Model file for the job. Use its own axes, mm. Give positions to 0.01 mm unless a question says otherwise; leave off trailing zeros. Loops run counter-clockwise (first coordinate to the right, second up) from the corner with the lowest first, then second, coordinate; pieces in that order, holes last. Notation, with made-up numbers: M 86,-12.5 L 90,-12.5 A30 ccw 90,18.5 Z; hole C -18,-1.5 d10. An arc over 180 degrees is marked long. Use CSV: the item, a comma, the result in double quotes. Start each with the question number.
(1) Slice it at C-C on y = 33.5. List the corners of the cut face in (x, z).
(2) Slice it at A-A on z = -55. List the corners of the cut face in (x, y).
(3) Flat gauge pins, fed straight in: P1, Ø4, axis at y = 39.24, z = 66.83, coming from the +X side; P2, Ø1, axis at x = 1, y = -15, coming from the -Z side; P3, Ø1, axis at x = -0.5, z = 19.5, coming from the -Y side; P4, Ø0.8, axis at x = 0, y = -22.5, coming from the +Z side. Where does each tip first touch, or does it go through?
(4) Slice it at B-B on x = 0.4. State how many separate pieces and enclosed holes the cut face has, and give its area (3 significant figures).
(5) Wall check: line 1 along Z through (x, y) = (0.5, 0); line 2 along Y through (x, z) = (-0.75, 0); line 3 along Y through (x, z) = (0.1, -22.5). Give the ranges that are in metal, low to high. Write a range as from..to.
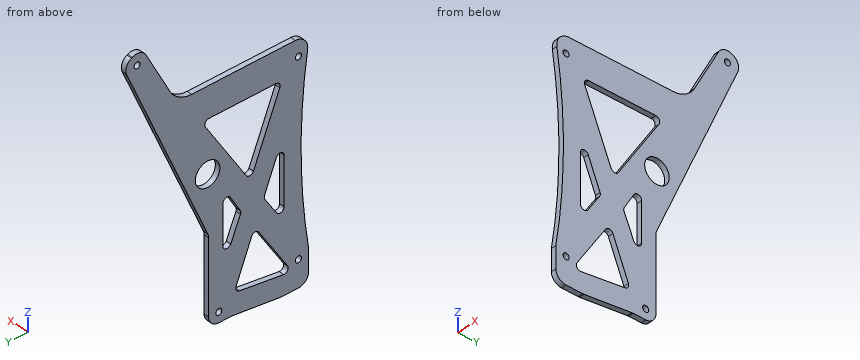
```python
from build123d import *

# Parameters (mm, degrees)
F0_R     = 1.5
F0_R_2   = 6
F1_DEPTH = 1.25


# Not quite as in the source:
# - ends of sketch curves that miss each other by under 0.0002 mm in the source are joined


with BuildPart() as f1:
    # F0 (on Right) → F1 (new body, symmetric)
    with BuildSketch(Plane.YZ):
        with BuildLine():
            ThreePointArc((-44.2615727709, 33.8276430339), (-41.0580126337, -11.4414374496), (-44.7615726272, -56.6723570594))
            Line((-44.7615726272, -56.6723570594), (-44.761573, -67.172357))
            ThreePointArc((-44.761573, -67.172357), (-43.2971069059, -70.7078909059), (-39.761573, -72.172357))
            Line((-39.761573, -72.172357), (-31.572862, -72.172357))
            ThreePointArc((-31.572862, -72.172357), (-31.2621746065, -72.1626949989), (-30.9526879578, -72.1337463374))
            Line((-30.9526879578, -72.1337463374), (-7.570458, -69.210968))
            ThreePointArc((-7.570458, -69.210968), (-7.2609713935, -69.1820190011), (-6.950284, -69.172357))
            Line((-6.950284, -69.172357), (-0.761573, -69.172357))
            ThreePointArc((-0.761573, -69.172357), (2.7739609059, -67.7078909059), (4.238427, -64.172357))
            Line((4.238427, -64.172357), (4.238427, -28.200354))
            ThreePointArc((4.238427, -28.200354), (4.340868282, -27.1934187471), (4.6439944414, -26.2277441895))
            Line((4.6439944414, -26.2277441895), (44.34607, 64.980308))
            ThreePointArc((44.34607, 64.980308), (44.4613498885, 68.6823868), (41.9976409775, 71.448035955))
            Line((41.9976409775, 71.448035955), (41.604729, 71.644492))
            ThreePointArc((41.604729, 71.644492), (37.8444305073, 71.9343641274), (34.9513503203, 69.5148688301))
            Line((34.9513503203, 69.5148688301), (23.120683, 47.205611))
            ThreePointArc((23.120683, 47.205611), (18.7052359642, 42.5450269916), (12.519138, 40.827643))
            Line((12.519138, 40.827643), (-38.220653, 40.827643))
            ThreePointArc((-38.220653, 40.827643), (-42.8437667533, 38.710714686), (-44.2615727709, 33.8276430339))
        make_face()
        with Locations((-39.761573, -59.172357)):
            Circle(F0_R, mode=Mode.SUBTRACT)
        with Locations((-0.761573, -64.172357)):
            Circle(F0_R, mode=Mode.SUBTRACT)
        with BuildLine():
            ThreePointArc((-9.2090828941, -56.8035819576), (-9.3358141293, -58.5495251427), (-10.7880590013, -59.5269519905))
            Line((-10.7880590013, -59.5269519905), (-32.462939, -62.56904))
            ThreePointArc((-32.462939, -62.56904), (-34.4234257272, -61.6697294934), (-34.4270410919, -59.5128209413))
            Line((-34.4270410919, -59.5128209413), (-20.357382, -37.45768))
            ThreePointArc((-20.357382, -37.45768), (-18.4841932611, -36.5420784276), (-16.8143035493, -37.7905298197))
            Line((-16.8143035493, -37.7905298197), (-9.2090828941, -56.8035819576))
        make_face(mode=Mode.SUBTRACT)
        with BuildLine():
            Line((-23.321557, -24.040332), (-29.08098, -32.967437))
            ThreePointArc((-29.08098, -32.967437), (-31.3267335557, -33.8016713068), (-32.761573, -31.883184))
            Line((-32.761573, -31.883184), (-32.761573, -8.557522))
            ThreePointArc((-32.761573, -8.557522), (-31.139788407, -6.5936092968), (-28.9046198941, -7.8147399576))
            Line((-28.9046198941, -7.8147399576), (-23.145197, -22.213297))
            ThreePointArc((-23.145197, -22.213297), (-23.0114029888, -23.1482412686), (-23.321557, -24.040332))
        make_face(mode=Mode.SUBTRACT)
        with BuildLine():
            ThreePointArc((-11.3658482669, -25.0957141144), (-11.5238882865, -24.1867752684), (-11.2571359352, -23.3036050376))
            Line((-11.2571359352, -23.3036050376), (-6.491151, -15.095519))
            ThreePointArc((-6.491151, -15.095519), (-4.2415517843, -14.1685784799), (-2.761573, -16.09979))
            Line((-2.761573, -16.09979), (-2.761573, -35.428508))
            ThreePointArc((-2.761573, -35.428508), (-4.3594410625, -37.387663406), (-6.5998629049, -36.2163469592))
            Line((-6.5998629049, -36.2163469592), (-11.3658482669, -25.0957141144))
        make_face(mode=Mode.SUBTRACT)
        with Locations((-39.761573, 32.827643)):
            Circle(F0_R, mode=Mode.SUBTRACT)
        with BuildLine():
            Line((5.800752, 22.759657), (-14.186435, -8.886721))
            ThreePointArc((-14.186435, -8.886721), (-16.0532082809, -9.8109940241), (-17.7292820906, -8.574103037))
            Line((-17.7292820906, -8.574103037), (-30.637673, 23.072275))
            ThreePointArc((-30.637673, 23.072275), (-30.4457341301, 24.9432737467), (-28.785804, 25.827643))
            Line((-28.785804, 25.827643), (4.109774, 25.827643))
            ThreePointArc((4.109774, 25.827643), (5.8613407009, 24.7930517696), (5.800752, 22.759657))
        make_face(mode=Mode.SUBTRACT)
        with Locations((4.738427, 0.827643)):
            Circle(F0_R_2, mode=Mode.SUBTRACT)
        with Locations((39.238427, 66.827643)):
            Circle(F0_R, mode=Mode.SUBTRACT)
    extrude(amount=F1_DEPTH, both=True)


solid = f1.part
```
Reply:
1,outline,"M -1.25,40.06 L 1.25,40.06 L 1.25,66.78 L -1.25,66.78 Z"
2,outline,"M -1.25,-44.5 L 1.25,-44.5 L 1.25,-31.55 L -1.25,-31.55 Z; M -1.25,-9.93 L 1.25,-9.93 L 1.25,4.24 L -1.25,4.24 Z"
3,P1,"stops at x = 1.25"
3,P2,"stops at z = -70.2"
3,P3,"stops at y = -42.55"
3,P4,"stops at z = 40.83"
4,separate pieces,"1"
4,enclosed holes,"9"
4,area,"5,040 mm^2"
5,line 1,"z = -69.11..-65.46, -62.88..-2.85, 4.51..13.58, 25.83..40.83"
5,line 2,"y = -41.21..-21.23, -8.57..-1.2, 10.68..16.06"
5,line 3,"y = -41.32..-32.76, -23.05..-10.79, -2.76..6.27"
